```python
from build123d import *

# Parameters (mm, degrees)
BOSS_EXTRUDE1_DEPTH = 40
BOSS_EXTRUDE5_DEPTH = 5
CUT_EXTRUDE2_DEPTH  = 19.5


with BuildPart() as part:
    # Sketch2 → Boss-Extrude1 (new body)
    with BuildSketch(Plane(origin=(0, 0, 0), x_dir=(1, 0, 0), z_dir=(0, 1, 0))):
        Polygon((52.905102206, -30.544775), (52.905102206, 30.544775), (0, 61.08955), (-52.905102206, 30.544775), (-52.905102206, -30.544775), (0, -61.08955), align=None)
        Polygon((45.905102206, -26.503323116), (45.905102206, 26.503323116), (0, 53.006646231), (-45.905102206, 26.503323116), (-45.905102206, -26.503323116), (0, -53.006646231), align=None, mode=Mode.SUBTRACT)
    extrude(amount=BOSS_EXTRUDE1_DEPTH)

    # Sketch7 → Boss-Extrude5 (add)
    with BuildSketch(Plane.XZ):
        Polygon((-49.405102206, 28.524049058), (-49.405102206, -28.524049058), (0, -57.048098116), (49.405102206, -28.524049058), (49.405102206, 28.524049058), (0, 57.048098116), align=None)
    extrude(amount=-BOSS_EXTRUDE5_DEPTH)

    # Sketch8 → Cut-Extrude2 (cut, symmetric)
    with BuildSketch(Plane.XY.offset(61)):
        with BuildLine():
            Line((3, 40), (3, 25))
            ThreePointArc((3, 25), (2.121320344, 22.878679656), (0, 22))
            ThreePointArc((0, 22), (-2.121320344, 22.878679656), (-3, 25))
            Line((-3, 25), (-3, 40))
            Line((-3, 40), (0, 40))
            Line((0, 40), (3, 40))
        make_face()
    extrude(amount=CUT_EXTRUDE2_DEPTH, both=True, mode=Mode.SUBTRACT)


solid = part.part
```
For this review, take the finished solid that the model builds, in its own axes (mm). A direction names the side the tool comes from. Give positions to 0.01 mm unless a question says otherwise; leave off trailing zeros. Write each loop counter-clockwise with the first axis right and the second up, starting at its lowest first coordinate (ties: lowest second). Pieces come first, ordered by that corner, then holes.
Item 1: Machinability: for faces 4 (the face through (0, 22, 56)), 5 (the face through (-45.905, 22, 0)), 6 (the face through (26.823, 19.72, -45.603)), which of the approach directions +Z, -Z, +X, -X, +Y, -Y give a long, thin tool a straight path to every point of the face, cutting with its end or side? Answer none if there is none.
Item 2: Insertion check: P1, Ø2, axis at x = -42, z = -6, coming from the +Y side; P2, Ø1.5, axis at x = -11, y = 35.5, coming from the +Z side; P3, Ø4, axis at x = -31.5, y = 5, coming from the +Z side. Each pin has a flat end and moves straight along its axis. Give the tip position at first contact, or say it passes through.
Item 3: Take a section at C-C (x = -4.5). Give the boundary of the cut face in (y, z), and give its area (3 significant figures).
Item 4: Take a section at A-A (z = -6). Give the boundary of the cut face in (x, y).
Item 5: Take a section at B-B (y = 31). Give the boundary of the cut face in (x, z), and give its area (3 significant figures).
Item 6: Wall thickness on probe 1 along X at (y, z) = (32.5, 22); probe 2 along Y at (x, z) = (19.5, 41); probe 3 along Z at (x, y) = (4, 9): over which ranges is each line inside the solid? List them lowest first.
Item 7: The part is to be moulded in two halves that separate along Z. For faces 1 (the face through (23.27, 22.26, -39.57)), 2 (the face through (52.905, 20, 0)), 3 (the face through (-26.823, 19.72, 45.603)), say which applies: +Z half, -Z half, draft (parallel to the pull), parting line (faces both ways), or undercut.
Established:
1. face 4: +Z, +Y
1. face 5: +Y
1. face 6: -Z, +X, +Y, -Y
2. P1: stops at y = 5
2. P2: stops at z = 55.17
2. P3: stops at z = 44.06
3. outline: (0, -58.49) - (40, -58.49) - (40, -50.41) - (5, -50.41) - (5, 50.41) - (40, 50.41) - (40, 58.49) - (0, 58.49) - close
3. area: 1,150 mm2
4. outline: (-52.91, 0) - (52.91, 0) - (52.91, 40) - (45.91, 40) - (45.91, 5) - (-45.91, 5) - (-45.91, 40) - (-52.91, 40) - close
5. outline: (-52.91, -30.54) - (0, -61.09) - (52.91, -30.54) - (52.91, 30.54) - (3, 59.36) - (3, 51.27) - (45.91, 26.5) - (45.91, -26.5) - (0, -53.01) - (-45.91, -26.5) - (-45.91, 26.5) - (-3, 51.27) - (-3, 59.36) - (-52.91, 30.54) - close
5. area: 2,350 mm2
6. probe 1: x = -52.91 to -45.91, 45.91 to 52.91
6. probe 2: y = 0 to 5
6. probe 3: z = -58.78 to -50.7, 50.7 to 58.78
7. face 1: undercut
7. face 2: draft
7. face 3: +Z half
